Design review of the part built by this model. Coordinates are the model's own, in mm. A direction names the side the tool comes from. Give positions to 0.01 mm unless a question says otherwise; leave off trailing zeros. Loops run counter-clockwise (first coordinate to the right, second up) from the corner with the lowest first, then second, coordinate; pieces in that order, holes last. Notation, with made-up numbers: (-33.5, -33) -> (-4.5, -33) arc R28 cw to (-4.5, -1) -> close; hole circle Ø8 at (22.5, 16). An arc over 180 degrees is marked (long way). Answer in a Markdown table with one row per item. Add a question column.
(1) Draft analysis for pull direction X (two halves, no side actions). For faces 1 (the flat face through (31.579, -0.014, -0.427)), 2 (the cylindrical face through (-2.45, -0.01, 0.08)), 3 (the flat face through (11, 1, 0)), state which applies: +X half, -X half, draft (parallel to the pull), parting line (faces both ways), or undercut.
(2) Consider section C-C on x = 0. Write out the cut boundary in (y, z).
(3) For faces 4 (the cylindrical face through (1.5, -6.42, 0.07)), 5 (the flat face through (9.201, -0.014, 1.563)), 6 (the flat face through (8.988, -0.014, -1.574)), list the 3-axis set-ups (+Z, -Z, +X, -X, +Y, -Y) from which the entire face can be reached by the end or side of a thin tool; tool diameter is ignored.
(4) Consider section D-D on x = 11.5. Write out the cut boundary in (y, z), then the cut area to 3 significant figures.
(5) For line 1 (X direction, y = -0.75, z = -2); line 2 (Z direction, x = 20, y = -0.15); line 3 (Y direction, x = 11, z = -0.75), list the stretches that pass through material, from the lowest coordinate up.
(6) Consider section B-B on y = -1.75. Write out the cut boundary in (x, z), then the cut area to 3 significant figures.
(7) Consider section A-A on x = 20. Write out the cut boundary in (y, z), then the cut area to 3 significant figures.
(8) For pin 1 (1.5 mm diameter, centred on x = 3.5, z = 1, fed in from -Y); pin 2 (4 mm diameter, centred on y = -4, z = -1.5, fed in from -X); pin 3 (5 mm diameter, centred on x = 31, y = -3, fed in from +Z), all flat-tipped, find the tip position at first contact; note any pin that passes through.
from build123d import *

# Parameters (mm, degrees)
F0_R     = 3.119034
F1_DEPTH = 1
F2_R     = 1.5
F3_DEPTH = 13


with BuildPart() as f1:
    # F0 (on Front) → F1 (new body, symmetric)
    with BuildSketch(Plane.XZ):
        with BuildLine():
            ThreePointArc((1.47637, -1.955206), (2.193126, -1.092106), (2.45, 0))
            ThreePointArc((2.45, 0), (2.193126, 1.092106), (1.47637, 1.955206))
            ThreePointArc((1.47637, 1.955206), (-2.45, 0), (1.47637, -1.955206))
        make_face()
        with BuildLine():
            ThreePointArc((1.47637, 1.955206), (2.193126, 1.092106), (2.45, 0))
            ThreePointArc((2.45, 0), (2.193126, -1.092106), (1.47637, -1.955206))
            Line((1.47637, -1.955206), (16.712802, -1.181905))
            ThreePointArc((16.712802, -1.181905), (16.506782, 0), (16.712802, 1.181905))
            Line((16.712802, 1.181905), (1.47637, 1.955206))
        make_face()
        with BuildLine():
            ThreePointArc((23.38997, 0.843016), (20.177065, 3.488727), (16.712802, 1.181905))
            ThreePointArc((16.712802, 1.181905), (16.506782, 0), (16.712802, -1.181905))
            ThreePointArc((16.712802, -1.181905), (20.177065, -3.488727), (23.38997, -0.843016))
            ThreePointArc((23.38997, -0.843016), (23.46731, -0.424657), (23.493218, 0))
            ThreePointArc((23.493218, 0), (23.46731, 0.424657), (23.38997, 0.843016))
        make_face()
        with Locations((20, 0)):
            Circle(F0_R, mode=Mode.SUBTRACT)
        with BuildLine():
            Line((40, 0), (23.38997, 0.843016))
            ThreePointArc((23.38997, 0.843016), (23.46731, 0.424657), (23.493218, 0))
            ThreePointArc((23.493218, 0), (23.46731, -0.424657), (23.38997, -0.843016))
            Line((23.38997, -0.843016), (40, 0))
        make_face()
    extrude(amount=F1_DEPTH, both=True)

    # F2 (on face) → F3 (join)
    with BuildSketch(Plane(origin=(0, 1, 0), x_dir=(-1, 0, 0), z_dir=(0, 1, 0))):
        Circle(F2_R)
    extrude(amount=-F3_DEPTH)


solid = f1.part
Values follow:
| question | item | result |
|---|---|---|
| 1 | face 1 | +X half |
| 1 | face 2 | undercut |
| 1 | face 3 | draft |
| 2 | outline | (-12, -1.5) -> (-1, -1.5) -> (-1, -2.45) -> (1, -2.45) -> (1, 2.45) -> (-1, 2.45) -> (-1, 1.5) -> (-12, 1.5) -> close |
| 3 | face 4 | -Y |
| 3 | face 5 | +Z, +Y, -Y |
| 3 | face 6 | -Z, +Y, -Y |
| 4 | outline | (-1, -1.45) -> (1, -1.45) -> (1, 1.45) -> (-1, 1.45) -> close |
| 4 | area | 5.79 mm2 |
| 5 | line 1 | -1.42 to 1.42, 17.14 to 17.61, 22.39 to 22.86 |
| 5 | line 2 | -3.49 to -3.12, 3.12 to 3.49 |
| 5 | line 3 | -1 to 1 |
| 6 | outline | circle Ø3 at (0, 0) |
| 6 | area | 7.07 mm2 |
| 7 | outline | (-1, -3.49) -> (1, -3.49) -> (1, -3.12) -> (-1, -3.12) -> close; (-1, 3.12) -> (1, 3.12) -> (1, 3.49) -> (-1, 3.49) -> close |
| 7 | area | 1.50 mm2 |
| 8 | pin 1 | y = -1 |
| 8 | pin 2 | x = -1.5 |
| 8 | pin 3 | z = 0.53 |
